Read the model definition and answer for the solid it produces. Units are mm, in the model's axes. Face numbers are marked on the shaded views. A direction names the side the tool comes from. Coordinates: 2 decimals unless noted, no trailing zeros. Write each loop counter-clockwise with the first axis right and the second up, starting at its lowest first coordinate (ties: lowest second). Pieces come first, ordered by that corner, then holes.
(1) Which of the six approach directions +Z, -Z, +X, -X, +Y, -Y give full straight-line access (tool end or side, diameter ignored) to the marked faces 1, 2, 3, 4 and 5?
(2) The part is cut by section A-A, the plane z = 1. Determine the outline of the cut face in (x, y).
(3) Given pin 1 (1.1 mm diameter, centred on x = 2, z = 0.5, fed in from -Y); pin 2 (2 mm diameter, centred on x = 4.5, z = 2, fed in from +Y); pin 3 (1.1 mm diameter, centred on x = 2, y = 0, fed in from +Z), each flat-ended and moving along its own axis, determine where each tip first touches the part or whether it passes through.
(4) Determine the mould class of the marked faces 6, 7, 8 and 9 for opening direction Z: pulls with the +Z half, pulls with the -Z half, needs draft (parallel to the pull), parting line crosses it, or undercut.
(5) The part is cut by section C-C, the plane x = 0. Determine the outline of the cut face in (y, z).
(6) The part is cut by section D-D, the plane x = 6. Determine the outline of the cut face in (y, z).
(7) The part is cut by section B-B, the plane y = 0.15. Determine the outline of the cut face in (x, z), and give its area (3 significant figures).
(8) Straight lines are drawn through the part: line 1 along X through (y, z) = (0.05, 1); line 2 along Y through (x, z) = (0, 0.65); line 3 along X through (y, z) = (-0.6, 1). For each, find the intervals that lie inside material, in ascending order.
```python
from build123d import *

# Parameters (mm, degrees)
SKETCH_1_R      = 1.5
SKETCH_1_R_2    = 1
EXTRUDE_1_DEPTH = 2
SKETCH_6_R      = 1.5
EXTRUDE_2_DEPTH = 1
EXTRUDE_3_DEPTH = 0.75
EXTRUDE_4_REACH = 8.98
SKETCH_10_W     = 1.5
SKETCH_10_H     = 1.5


with BuildPart() as part:
    # Sketch 1 → Extrude 1 (new body)
    with BuildSketch(Plane.XY):
        Circle(SKETCH_1_R)
        Circle(SKETCH_1_R_2, mode=Mode.SUBTRACT)
    extrude(amount=EXTRUDE_1_DEPTH)

    # Sketch 8 → Extrude 3 (add, symmetric)
    with BuildSketch(Plane.XY.offset(1)):
        with BuildLine():
            Line((1.299038106, 0.75), (1.771810874, 0.75))
            Line((1.771810874, 0.75), (1.771810874, -0.75))
            Line((1.771810874, -0.75), (1.299038106, -0.75))
            ThreePointArc((1.299038106, -0.75), (1.5, 0), (1.299038106, 0.75))
        make_face()
    extrude(amount=EXTRUDE_3_DEPTH, both=True)


with BuildPart() as body_2:
    # Sketch 6 → Extrude 2 (new, symmetric)
    with BuildSketch(Plane(origin=(0, 0, 0), x_dir=(1, 0, 0), z_dir=(0, 1, 0))):
        with BuildLine():
            Line((6.372879371, 0.56), (7.074881195, 0.56))
            ThreePointArc((7.074881195, 0.56), (5.121320344, -3.5), (3.167759492, 0.56))
            Line((3.167759492, 0.56), (3.869761316, 0.56))
            ThreePointArc((3.869761316, 0.56), (5.121320344, 1), (6.372879371, 0.56))
        make_face()
        with Locations(Location((5.121320344, -1, 0), (0, 0, 270))):
            Circle(SKETCH_6_R, mode=Mode.SUBTRACT)
    extrude(amount=EXTRUDE_2_DEPTH, both=True)

    # Sketch 10 → Extrude 4 (add, up to next)
    with BuildSketch(Plane(origin=(1.771810874, 0, 0), x_dir=(0, 0, -1), z_dir=(1, 0, 0)), mode=Mode.PRIVATE) as extrude_4_sk1:
        with Locations((-1, 0)):
            Rectangle(SKETCH_10_W, SKETCH_10_H)
    extrude_4_tool1 = extrude(extrude_4_sk1.sketch, amount=EXTRUDE_4_REACH, mode=Mode.PRIVATE) - body_2.part

    add(part.part)  # Extrude 4 merges part
    add(extrude_4_tool1.solids().sort_by_distance((1.771811, 0, 1))[0])


solid = body_2.part
```
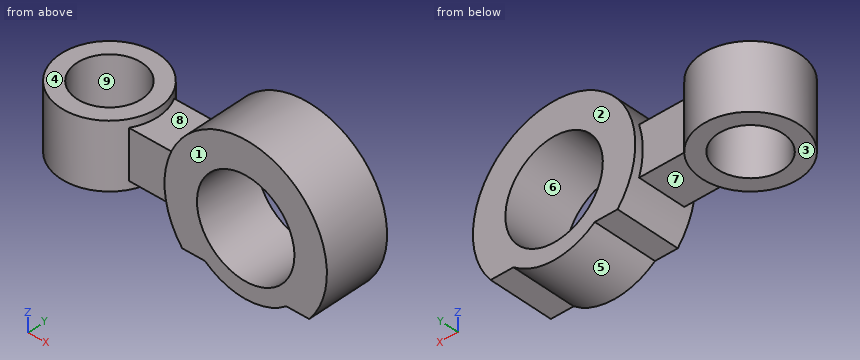
Computed:
1. face 1: +Z, -Z, +X, -Y
1. face 2: +Z, -Z, +X, +Y
1. face 3: -Z, -X, +Y, -Y
1. face 4: +Z, -X, +Y, -Y
1. face 5: -Z, +Y, -Y
2. outline: (1.3, -0.75) - (2.62, -0.75) - (2.62, -1) - (3.62, -1) - (3.62, 1) - (2.62, 1) - (2.62, 0.75) - (1.3, 0.75) arc R1.5 ccw (long way) to start; (6.62, -1) - (7.62, -1) - (7.62, 1) - (6.62, 1) - close; hole circle Ø2 at (0, 0)
3. pin 1: stops at y = -0.75
3. pin 2: stops at y = 1
3. pin 3: stops at z = 2
4. face 6: undercut
4. face 7: pulls with the -Z half
4. face 8: pulls with the +Z half
4. face 9: needs draft
5. outline: (-1.5, 0) - (-1, 0) - (-1, 2) - (-1.5, 2) - close; (1, 0) - (1.5, 0) - (1.5, 2) - (1, 2) - close
6. outline: (-1, -0.8) - (1, -0.8) - (1, -0.22) - (-1, -0.22) - close; (-1, 2.22) - (1, 2.22) - (1, 3.34) - (-1, 3.34) - close
7. outline: (-1.49, 0) - (-0.99, 0) - (-0.99, 2) - (-1.49, 2) - close; (0.99, 0) - (1.49, 0) - (1.49, 0.25) - (2.74, 0.25) arc R2.5 ccw to (3.17, -0.56) - (3.87, -0.56) arc R2 ccw to (6.37, -0.56) - (7.07, -0.56) arc R2.5 ccw (long way) to (2.74, 1.75) - (1.49, 1.75) - (1.49, 2) - (0.99, 2) - close; hole circle Ø3 at (5.12, 1)
7. area: 14.5 mm2
8. line 1: x = -1.5 to -1, 1 to 3.62, 6.62 to 7.62
8. line 2: y = -1.5 to -1, 1 to 1.5
8. line 3: x = -1.37 to -0.8, 0.8 to 3.62, 6.62 to 7.62
